Verification items for the finished model (mm, model axes). A direction names the side the tool comes from. Coordinates: 2 decimals unless noted, no trailing zeros. Write each loop counter-clockwise with the first axis right and the second up, starting at its lowest first coordinate (ties: lowest second). Pieces come first, ordered by that corner, then holes.
```python
from build123d import *

# Parameters (mm, degrees)
CROQUIS1_W              = 32
CROQUIS1_H              = 13.5
CROQUIS1_R              = 2.6
CROQUIS1_R_2            = 1
SALIENTE_EXTRUIR1_DEPTH = 1
SALIENTE_EXTRUIR2_DEPTH = 1


with BuildPart() as part:
    # Croquis1 → Saliente-Extruir1 (new body)
    with BuildSketch(Plane.XY):
        with Locations((16, -6.75)):
            Rectangle(CROQUIS1_W, CROQUIS1_H)
        with Locations((8.1, -6.75)):
            Circle(CROQUIS1_R, mode=Mode.SUBTRACT)
        with Locations((29, -6.75)):
            Circle(CROQUIS1_R_2, mode=Mode.SUBTRACT)
    extrude(amount=SALIENTE_EXTRUIR1_DEPTH)

    # Croquis2 → Saliente-Extruir2 (add)
    with BuildSketch(Plane(origin=(0, 0, 0), x_dir=(1, 0, 0), z_dir=(0, 1, 0))):
        Polygon((1.571524395, -1), (13.606050016, -3.5), (28.926741078, -1), align=None)
    saliente_extruir2 = extrude(amount=-SALIENTE_EXTRUIR2_DEPTH)

    # Simetría1: Saliente-Extruir2 across plane
    add(saliente_extruir2.mirror(Plane.ZX.offset(-6.75)))


solid = part.part
```
1. Sectioned sample at D-D, the plane x = 8.1. Record the boundary of the cut face in (y, z).
2. Draft check along Y on faces 3 (the flat face through (16, -13.5, 1)), 4 (the flat face through (15, -12.5, 2)), 5 (the flat face through (0, -6.8, 0.5)). Enter one of: pulls with the +Y half, pulls with the -Y half, needs draft (parallel to the pull), parting line crosses it, or undercut.
3. Material ranges on L1, parallel to Y at x = 29, z = 0.7; L2, parallel to Y at x = 8.1, z = 0.35; L3, parallel to Z at x = 7, y = -3, recorded low to high.
4. Gauge pin test, flat ends, axial feed: P1, Ø1.5, axis at x = 15.5, y = -6, coming from the +Z side; P2, Ø3, axis at x = 8.1, y = -6.75, coming from the +Z side. Record the tip position at first contact, or that the pin passes through.
5. Sectioned sample at A-A, the plane y = -6.75. Record the boundary of the cut face in (x, z), and give its area (3 significant figures).
6. Tool access check on faces 1 (the flat face through (32, -6.8, 0.5)), 2 (the flat face through (15, -1, 2)). Record the directions out of +Z, -Z, +X, -X, +Y, -Y that give a thin tool (end or side, any length) a straight path to the whole face; none if there is none.
7. Sectioned sample at B-B, the plane z = 2.35. Record the boundary of the cut face in (x, y), and give its area (3 significant figures).
8. Sectioned sample at C-C, the plane y = -5. Record the boundary of the cut face in (x, z), and give its area (3 significant figures).
Outcome:
1. outline: (-13.5, 0) - (-9.35, 0) - (-9.35, 1) - (-12.5, 1) - (-12.5, 2.36) - (-13.5, 2.36) - close; (-4.15, 0) - (0, 0) - (0, 2.36) - (-1, 2.36) - (-1, 1) - (-4.15, 1) - close
2. face 3: pulls with the -Y half
2. face 4: undercut
2. face 5: needs draft
3. L1: y = -13.5 to -7.75, -5.75 to 0
3. L2: y = -13.5 to -9.35, -4.15 to 0
3. L3: z = 0 to 1
4. P1: stops at z = 1
4. P2: passes through
5. outline: (0, 0) - (5.5, 0) - (5.5, 1) - (0, 1) - close; (10.7, 0) - (28, 0) - (28, 1) - (10.7, 1) - close; (30, 0) - (32, 0) - (32, 1) - (30, 1) - close
5. area: 24.8 mm2
6. face 1: +Z, -Z, +X, +Y, -Y
6. face 2: +Z, +X, -X
7. outline: (8.07, -13.5) - (20.65, -13.5) - (20.65, -12.5) - (8.07, -12.5) - close; (8.07, -1) - (20.65, -1) - (20.65, 0) - (8.07, 0) - close
7. area: 25.2 mm2
8. outline: (0, 0) - (6.18, 0) - (6.18, 1) - (0, 1) - close; (10.02, 0) - (32, 0) - (32, 1) - (10.02, 1) - close
8. area: 28.2 mm2
